Check sheet for the modelled part. Datum: model origin and axes. Units: mm. A direction names the side the tool comes from. Round coordinates to 2 decimals unless told otherwise and drop trailing zeros. Loops run counter-clockwise (first coordinate to the right, second up) from the corner with the lowest first, then second, coordinate; pieces in that order, holes last. Notation, with made-up numbers: (55.25, 10.25) - (113.25, 10.25) arc R30 ccw to (113.25, 46.25) - close; hole circle Ø3 at (49, 76). An arc over 180 degrees is marked (long way). Return JSON: item names as keys, results as strings.
from build123d import *

# Parameters (mm, degrees)
PAD_DEPTH = 50


with BuildPart() as part:
    # Sketch → Pad (new body)
    with BuildSketch(Plane.XY):
        with BuildLine():
            ThreePointArc((-34.7, 14), (-30.7, 18), (-34.7, 22))
            Line((-38.7, 22), (-34.7, 22))
            ThreePointArc((-38.7, 22), (-40.114214, 21.414214), (-40.7, 20))
            Line((-40.7, 0), (-40.7, 20))
            Line((0, 0), (-40.7, 0))
            Line((40.7, 0), (0, 0))
            Line((40.7, 20), (40.7, 0))
            ThreePointArc((40.7, 20), (40.114214, 21.414214), (38.7, 22))
            Line((34.7, 22), (38.7, 22))
            ThreePointArc((34.7, 22), (30.7, 18), (34.7, 14))
            Line((34.7, 14), (36.7, 14))
            Line((36.7, 14), (36.7, 8))
            Line((-36.7, 8), (36.7, 8))
            Line((-36.7, 14), (-36.7, 8))
            Line((-34.7, 14), (-36.7, 14))
        make_face()
    extrude(amount=PAD_DEPTH)


solid = part.part
Q1. Sectioned sample at A-A (y = 12). Enter the section's corners in (x, z).
Answer key:
{"outline": "(-40.7, 0) - (-36.7, 0) - (-36.7, 50) - (-40.7, 50) - close; (36.7, 0) - (40.7, 0) - (40.7, 50) - (36.7, 50) - close"}
Q2. Scan lines: probe 1 along X at (y, z) = (13.75, 33); probe 2 along X at (y, z) = (18, 37.5); probe 3 along Y at (x, z) = (-36.5, 48). Record each from-to range of solid material in increasing order. Write a range as [from, to].
Answer key:
{"probe 1": "x = [-40.7, -36.7], [36.7, 40.7]", "probe 2": "x = [-40.7, -30.7], [30.7, 40.7]", "probe 3": "y = [0, 8], [14, 22]"}
Q3. Sectioned sample at B-B (z = 35). Enter the section's corners in (x, y).
Answer key:
{"outline": "(-40.7, 0) - (40.7, 0) - (40.7, 20) arc R2 ccw to (38.7, 22) - (34.7, 22) arc R4 ccw to (34.7, 14) - (36.7, 14) - (36.7, 8) - (-36.7, 8) - (-36.7, 14) - (-34.7, 14) arc R4 ccw to (-34.7, 22) - (-38.7, 22) arc R2 ccw to (-40.7, 20) - close"}
Q4. Depth check by flat-ended pin: P1, Ø0.6, axis at x = 36, z = 27.5, coming from the -Y side; P2, Ø12, axis at x = -21, z = 42, coming from the +Y side. Enter the tip coordinate at first touch or a pass-through.
Answer key:
{"P1": "stops at y = 0", "P2": "stops at y = 8"}
Q5. Draft check along Y on faces 3 (the face through (-40.1, 21.43, 24.65)), 4 (the face through (-30.7, 17.9, 24.6)), 5 (the face through (40.7, 10, 25)). Enter one of: released by +Y, released by -Y, zero draft, split by the parting line, or undercut.
Answer key:
{"face 3": "released by +Y", "face 4": "undercut", "face 5": "zero draft"}
Q6. Tool access check on faces 1 (the face through (-37, 22, 25)), 2 (the face through (30.7, 18.1, 24.6)). Record the directions out of +Z, -Z, +X, -X, +Y, -Y that give a thin tool (end or side, any length) a straight path to the whole face; none if there is none.
Answer key:
{"face 1": "+Z, -Z, +X, -X, +Y", "face 2": "+Z, -Z"}
Q7. Sectioned sample at C-C (x = 20.5). Enter the section's corners in (y, z), plus the area to 3 significant figures.
Answer key:
{"outline": "(0, 0) - (8, 0) - (8, 50) - (0, 50) - close", "area": "400 mm²"}
